Design review of the part built by this model. Coordinates are the model's own, in mm. A direction names the side the tool comes from. Give positions to 0.01 mm unless a question says otherwise; leave off trailing zeros. Use one line per item in the form item = value. Start each with the question number.
from build123d import *

# Parameters (mm, degrees)
F2_R            = 2.5
F3_R            = 0.25
F4_SIZE         = 1
F5_SIZE         = 3
F7_D            = 7.5
F7_COPIES_COUNT = 8
F8_W            = 5
F8_H            = 12.3844173994
F10_W           = 3.9803426395
F10_H           = 3


# Not quite as in the source:
# - a pattern or mirror of a feature is missing from the dataset's text; its kind, count and spacing are read off the source's solid


with BuildPart() as f1:
    # F0 (on Top) → F1 (revolve)
    with BuildSketch(Plane.XY):
        Polygon((70, 15), (35, 15), (35, 40), (20, 40), (20, 30), (23, 30), (23, 25), (20, 25), (20, 0), (70, 0), align=None)
    revolve(axis=Axis((0, 48.9874315186, 0), (0, 1, 0)))

    # F2
    f2_edges = [f1.edges().sort_by_distance(p)[0] for p in [
        (-35, 15, 0),
    ]]
    fillet(f2_edges, radius=F2_R)

    # F3
    f3_edges = [f1.edges().sort_by_distance(p)[0] for p in [
        (-23, 30, 0),
        (-23, 25, 0),
    ]]
    fillet(f3_edges, radius=F3_R)

    # F4
    f4_edges = [f1.edges().sort_by_distance(p)[0] for p in [
        (-20, 0, 0),
    ]]
    chamfer(f4_edges, length=F4_SIZE)

    # F5
    f5_edges = [f1.edges().sort_by_distance(p)[0] for p in [
        (-70, 0, 0),
    ]]
    chamfer(f5_edges, length=F5_SIZE)

    # F7 (through all)
    with Locations(Plane(origin=(0, 15, 0), x_dir=(-1, 0, 0), z_dir=(0, 1, 0))):
        with Locations((0, -48)):
            f7 = Hole(F7_D / 2)

    # F7_copies: F7 ×8 about axis
    f7_copies_axis = Axis((0, 0, 0), (0, 1, 0))
    for i in range(1, F7_COPIES_COUNT):
        add(f7.rotate(f7_copies_axis, i * 360 / F7_COPIES_COUNT), mode=Mode.SUBTRACT)

    # F8 (on Right) → F9 (revolve, cut)
    with BuildSketch(Plane.YZ):
        with Locations((31.5, 39.1922086997)):
            Rectangle(F8_W, F8_H)
    revolve(axis=Axis((0, 33.8349905132, 0), (0, 1, 0)), mode=Mode.SUBTRACT)

    # F10 (on Right) → F11 (revolve, cut)
    with BuildSketch(Plane.YZ):
        with Locations((40.9901713197, 29.5)):
            Rectangle(F10_W, F10_H)
    revolve(axis=Axis((0, 26.3936025676, 0), (0, 1, 0)), mode=Mode.SUBTRACT)


solid = f1.part
1. Draft analysis for pull direction X (two halves, no side actions). For faces 1 (the cylindrical face through (-28, 37, 21)), 2 (the flat face through (-27.4, 39, 7)), 3 (the flat face through (-20.9, 40, 23.2)), state which applies: pulls with the +X half, pulls with the -X half, needs draft (parallel to the pull), parting line crosses it, or undercut.
2. We need section A-A (y = 9). Give the number of separate pieces and of enclosed holes in the cut face, and give its area (3 significant figures).
3. To check wall thickness, follow L1, parallel to Z at x = 0, y = 5.5; L2, parallel to X at y = 26, z = 0; L3, parallel to Z at x = -11, y = 36.5. State the ranges of each line that lie inside material, in increasing order.
4. Clearance check with flat-ended pins moving along their axes: pin 1 Ø7 at (x, z) = (48, 0) entering from -Y; pin 2 Ø8.5 at (x, z) = (33.94, 33.94) entering from +Y; pin 3 Ø6 at (y, z) = (20.5, -2.5) entering from -X; pin 4 Ø1 at (y, z) = (29, -4.5) entering from +X. State where each tip first meets the part, or that it passes through.
5. For faces 4 (the flat face through (30, 15, 30)), 5 (the conical face through (-14.565, 0.188, 65.59)), 6 (the flat face through (1.6, 25, 20.1)), list the 3-axis set-ups (+Z, -Z, +X, -X, +Y, -Y) from which the entire face can be reached by the end or side of a thin tool; tool diameter is ignored.
Answer block:
q1.face_1 = parting line crosses it
q1.face_2 = undercut
q1.face_3 = needs draft
q2.separate_pieces = 1
q2.enclosed_holes = 9
q2.area = 13,800 mm^2
q3.L1 = -70 to -51.75, -44.25 to -20, 20 to 44.25, 51.75 to 70
q3.L2 = -35 to -23, 23 to 35
q3.L3 = -33.23 to -16.7, 16.7 to 33.23
q4.pin_1 = through
q4.pin_2 = 15
q4.pin_3 = -35
q4.pin_4 = 34.77
q5.face_4 = +Y
q5.face_5 = -Y
q5.face_6 = none
